Geometry: see drawing. Coordinates: mm, zero at the bounding-box minimum. Coordinates: 2 decimals unless noted, no trailing zeros. Order: outer loops, then holes, each group sorted by start corner. A loop starts at its lowest first (then second) coordinate and runs counter-clockwise, first axis right, second up.
Item 1: Mould query, pull axis Y, two halves, no side actions, for the marked faces 1, 2 and 3. Classes: released by +Y, released by -Y, zero draft, split by the parting line, or undercut.
Item 2: Ray query, line 1 (Y direction, x = 69.5, z = 91.5); line 2 (X direction, y = 11.5, z = 65) (1 decimal); line 3 (Z direction, x = 152.5, y = 69.5). Return the intervals inside material, ascending.
Item 3: Section A-A on z = 127. Return the cut outline in (x, y), then the cut area to 3 significant figures.
Item 4: Section D-D on x = 69.85. Return the cut outline in (y, z).
Item 5: Section B-B on y = 45.5. Return the cut outline in (x, z).
Item 6: Section C-C on x = 115.5. Return the cut outline in (y, z), then the cut area to 3 significant figures.
Item 7: Contact query for flat-ended pins moving along their axis: P1, Ø15, axis at y = 129, z = 168.5, coming from the +X side; P2, Ø5.5, axis at y = 5, z = 169.5, coming from the +X side; P3, Ø10, axis at x = 70, y = 33, coming from the +Z side. Output: stop coordinate, or through.
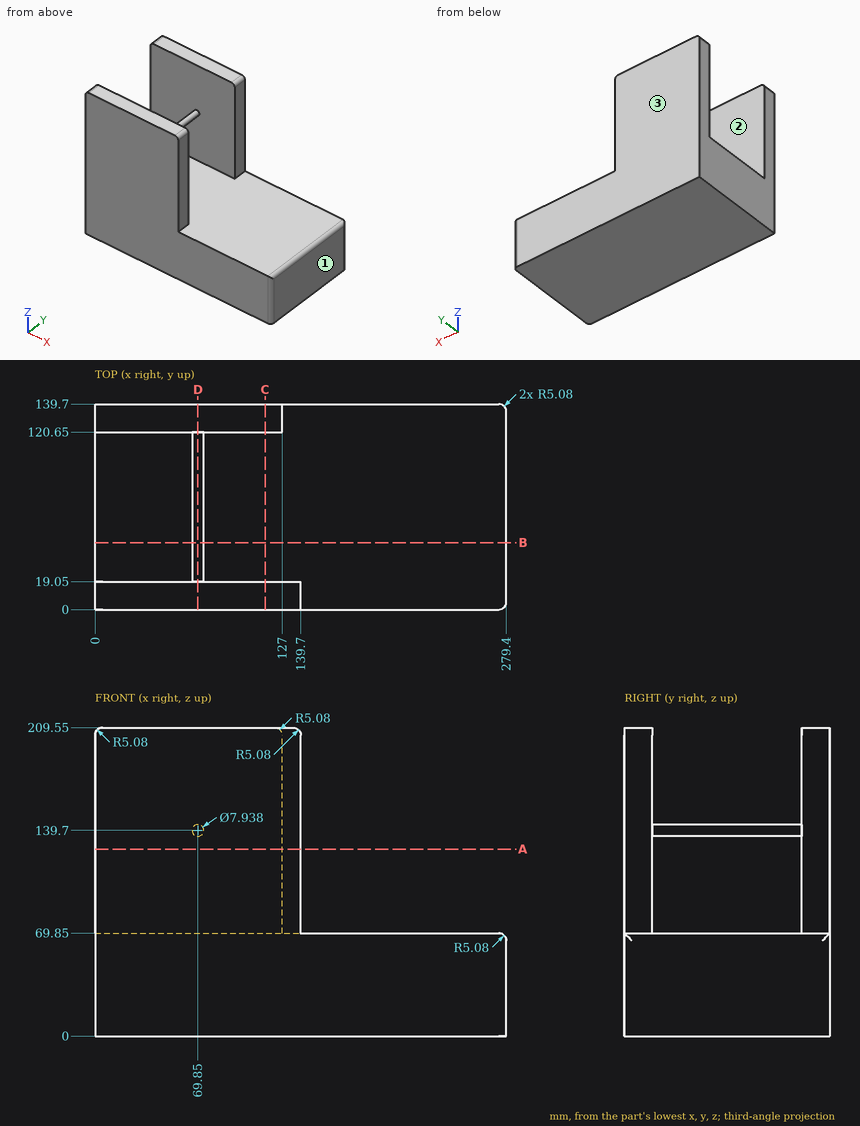
Answer list:
1. face 1: zero draft
1. face 2: undercut
1. face 3: released by +Y
2. line 1: y = 0 to 19.05, 120.65 to 139.7
2. line 2: x = 0 to 279.4
2. line 3: z = 0 to 69.85
3. outline: (0, 0) - (139.7, 0) - (139.7, 19.05) - (0, 19.05) - close; (0, 120.65) - (127, 120.65) - (127, 139.7) - (0, 139.7) - close
3. area: 5,080 mm2
4. outline: (0, 0) - (139.7, 0) - (139.7, 209.55) - (120.65, 209.55) - (120.65, 143.67) - (19.05, 143.67) - (19.05, 209.55) - (0, 209.55) - close; hole (19.05, 69.85) - (120.65, 69.85) - (120.65, 135.73) - (19.05, 135.73) - close
5. outline: (0, 0) - (279.4, 0) - (279.4, 64.77) arc R5.08 ccw to (274.32, 69.85) - (0, 69.85) - close; circle Ø7.94 at (69.85, 139.7)
6. outline: (0, 0) - (139.7, 0) - (139.7, 209.55) - (120.65, 209.55) - (120.65, 69.85) - (19.05, 69.85) - (19.05, 209.55) - (0, 209.55) - close
6. area: 15,100 mm2
7. P1: stops at x = 127
7. P2: stops at x = 139.7
7. P3: stops at z = 143.67
